Solid Edge part; units mm, degrees
sketch "Sketch1" plane through (0, 0, 0) normal (0, 0, 1) x (1, 0, 0)
  line L0 (-5, -5) -> (5, -5)
  line L1 (5, -5) -> (5, 5)
  line L2 (5, 5) -> (10, 5)
  line L3 (10, 5) -> (10, 14)
  line L4 (10, 14) -> (7, 14)
  line L5 (7, 14) -> (7, 8)
  line L6 (7, 8) -> (-7, 8)
  line L7 (-7, 8) -> (-7, 14)
  line L8 (-7, 14) -> (-10, 14)
  line L9 (-10, 14) -> (-10, 5)
  line L10 (-10, 5) -> (-5, 5)
  line L11 (-5, 5) -> (-5, -5)
  dimension "D1" = 5
  dimension "D2" = 5
  dimension "D3" = 5
  dimension "D4" = 10
  dimension "D5" = 7
  dimension "D6" = 7
extrude "Ajout_matière_1" add sketch "Sketch1" along normal mid plane 20
hole "Perçage_1" at (0, 0, 10) direction (0, 0, -1) diameter 4.459 end up to next
hole "Perçage_2" at (10, 11, 7) direction (-1, 0, 0) diameter 3 end through all
hole "Hole1" at (10, 11, 0) direction (-1, 0, 0) diameter 3 end through all
hole "Hole2" at (10, 11, -7) direction (-1, 0, 0) diameter 3 end through all
hole "Perçage_5" at (5, 0, 0) direction (-1, 0, 0) diameter 4 end up to next
chamfer "Chanfrein_1" distance 1 angle 45 6 edges at (10, 14, 0) (10, 5, 0) (-10, 14, 0) (-10, 5, 0) (-5, -5, 0) (5, -5, 0)
sketch "Sketch2" plane through (0, 8, 0) normal (0, 1, 0) x (0, 0, -1)
  line L0 (-4.5, 6) -> (-2.5, 6)
  line L1 (-2.5, 6) -> (-2.5, -6)
  line L2 (-2.5, -6) -> (-4.5, -6)
  line L3 (-4.5, -6) -> (-4.5, 6)
  line L4 (2.5, -6) -> (4.5, -6)
  line L5 (4.5, -6) -> (4.5, 6)
  line L6 (4.5, 6) -> (2.5, 6)
  line L7 (2.5, 6) -> (2.5, -6)
  dimension "D1" = 2.5
  dimension "D2" = 2.5
extrude "Ajout_matière_2" add sketch "Sketch2" along normal blind 2 and the other way blind 0.7497
properties material "Aluminium AU4G, 2024_T4"
Model file for the job. Use its own axes, mm. A direction names the side the tool comes from. Give positions to 0.01 mm unless a question says otherwise; leave off trailing zeros. Loops run counter-clockwise (first coordinate to the right, second up) from the corner with the lowest first, then second, coordinate; pieces in that order, holes last.
Item 1: Slice it at D-D (x = 0). Write the cut outline in (y, z), plus the area to 3 significant figures.
Check values:
outline: (-5, -10) - (-2.23, -10) - (-2.23, 10) - (-5, 10) - close; (2.23, -10) - (8, -10) - (8, -4.5) - (10, -4.5) - (10, -2.5) - (8, -2.5) - (8, 2.5) - (10, 2.5) - (10, 4.5) - (8, 4.5) - (8, 10) - (2.23, 10) - close
area: 179 mm2
Item 2: Drill centre lines: line 1 along Z through (x, y) = (9.05, 11); line 2 along Y through (x, z) = (-7.55, 0); line 3 along Y through (x, z) = (5.75, -7). Where is each one in solid material? Low to high.
Check values:
line 1: z = -10 to -8.5, -5.5 to -1.5, 1.5 to 5.5, 8.5 to 10
line 2: y = 5 to 9.5, 12.5 to 14
line 3: y = 5 to 8
Item 3: Slice it at C-C (z = 0). Give the number of separate pieces and of enclosed holes in the cut face, plus the area to 3 significant figures.
Check values:
separate pieces: 3
enclosed holes: 0
area: 147 mm2
Item 4: Drop flat-ended pins along their axis: P1, Ø5, axis at x = 4.5, z = -7, coming from the -Y side; P2, Ø2.5, axis at y = 11, z = 7, coming from the +X side (3 decimals); P3, Ø3, axis at x = -8, z = -3.5, coming from the -Y side; P4, Ø0.6, axis at x = -0.5, y = 9.5, coming from the -Z side. Give the stop position or say it passes through.
Check values:
P1: stops at y = -5
P2: passes through
P3: stops at y = 5
P4: stops at z = -4.5
Item 5: Which spindle directions (+Z, -Z, +X, -X, +Y, -Y) get a long thin tool onto all of the face, cutting with end or side? Do faces 1 (the face through (-7, 5, 0)), 2 (the face through (-6, 9, 4)), 3 (the face through (-8.48, 11.07, -5.5)), 4 (the face through (0, 9, -4.5)). Say none if no direction does.
Check values:
face 1: +Z, -Z, -X, -Y
face 2: +Z, -Z, +Y
face 3: +X, -X
face 4: -Z, +Y
Item 6: Slice it at A-A (z = 7). Write the cut outline in (x, y), plus the area to 3 significant figures.
Check values:
outline: (-10, 6) - (-9, 5) - (-5, 5) - (-5, -4) - (-4, -5) - (4, -5) - (5, -4) - (5, 5) - (9, 5) - (10, 6) - (10, 9.5) - (7, 9.5) - (7, 8) - (-7, 8) - (-7, 9.5) - (-10, 9.5) - close; (-10, 12.5) - (-7, 12.5) - (-7, 14) - (-9, 14) - (-10, 13) - close; (7, 12.5) - (10, 12.5) - (10, 13) - (9, 14) - (7, 14) - close; hole circle Ø4.46 at (0, 0)
area: 159 mm2
Item 7: Slice it at B-B (y = 0). Write the cut outline in (x, z), plus the area to 3 significant figures.
Check values:
outline: (-5, -10) - (-2.23, -10) - (-2.23, 10) - (-5, 10) - close; (2.23, -10) - (5, -10) - (5, -2) - (2.23, -2) - close; (2.23, 2) - (5, 2) - (5, 10) - (2.23, 10) - close
area: 99.7 mm2
Item 8: Mould opens along X. For faces 5 (the face through (0, 9, 4.5)), 6 (the face through (7, 5, 0)), 7 (the face through (-9.5, 13.5, -0.1)) say: +X half, -X half, draft (parallel to the pull), parting line (faces both ways), or undercut.
Check values:
face 5: undercut
face 6: draft
face 7: -X half
